Work out the finished part from the listing and answer in its coordinate system (mm). A direction names the side the tool comes from. Coordinates: 2 decimals unless noted, no trailing zeros. Order: outer loops, then holes, each group sorted by start corner. A loop starts at its lowest first (then second) coordinate and runs counter-clockwise, first axis right, second up. Notation, with made-up numbers: (29.25, -18) - (86.25, -18) arc R32 cw to (86.25, 20) - close; hole circle Ø2 at (76, 37.25). An arc over 180 degrees is marked (long way). Answer as a JSON object with one key per item and string values. Group by question number.
1) Find the intervals of material crossed by line 1 along X through (y, z) = (-14, -44); line 2 along X through (y, z) = (-0.5, -89.5); line 3 along Z through (x, y) = (51, 0), in increasing order.
2) Section A-A (z = -85) is taken. Count the separate pieces of the cut face and the enclosed holes in it, plus the area to 3 significant figures.
3) The mould has two halves that part along Z. Classify faces 6 (the face through (52, -8, -48)), 7 (the face through (66.667, 2, -86)), 8 (the face through (-70.388, -7.598, -95.496)): released by +Z, released by -Z, zero draft, split by the parting line, or undercut.
4) This flat-tipped pin is pushed along its axis until it touches: P1, Ø1.1, axis at x = -67.5, z = -25.5, coming from the -Y side. Where does it stop, or does it pass through?
5) Section D-D (y = -16) is taken. Give the vertices of the cut face in (x, z), plus the area to 3 significant figures.
6) Section B-B (x = 61) is taken. Give the vertices of the cut face in (y, z), plus the area to 3 significant figures.
7) A tool of negligible diameter and unlimited length cuts with its end or side. For faces 1 (the face through (-53.5, -9, -49)), 2 (the face through (71.814, -8, -49)), 3 (the face through (-52, -8, -48)), 4 (the face through (-66.667, 2, -12)), 5 (the face through (-70.311, -7.598, -1.426)), from which of +Z, -Z, +X, -X, +Y, -Y can it reach the whole face along a straight path? Write none if from no direction.
from build123d import *
from build123d.topology import SkipClean

# Parameters (mm, degrees)
CROQUIS1_W              = 114
CROQUIS1_H              = 34.2
SALIENTE_EXTRUIR1_DEPTH = 97
VACIADO1_T              = -5
SALIENTE_EXTRUIR2_DEPTH = 97
CORTAR_EXTRUIR1_REACH   = 128.031
CROQUIS3_W              = 13.814275766
CROQUIS3_H              = 40
REDONDEO2_R             = 5
CROQUIS6_W              = 12.3
CROQUIS6_H              = 10.4
CORTAR_EXTRUIR3_DEPTH   = 124.459670354
SALIENTE_EXTRUIR3_DEPTH = 97
CROQUIS8_W              = 13.814275766
CROQUIS8_H              = 40
CORTAR_EXTRUIR4_DEPTH   = 127.030661617
CROQUIS9_W              = 104
CROQUIS9_H              = 87
CORTAR_EXTRUIR5_DEPTH   = 10
CORTAR_EXTRUIR6_START   = -33.316303
CROQUIS11_W             = 1.5
CROQUIS11_H             = 39.999512223
CROQUIS11_H_2           = 40
CORTAR_EXTRUIR6_DEPTH   = 33.316303
CORTAR_EXTRUIR7_START   = -33.316303
CROQUIS13_W             = 15.314275766
CROQUIS13_H             = 4.5
CORTAR_EXTRUIR7_DEPTH   = 33.316303


with BuildPart() as part:
    # Croquis1 → Saliente-Extruir1 (new body)
    with BuildSketch(Plane.XY):
        with Locations((0, -8.9)):
            Rectangle(CROQUIS1_W, CROQUIS1_H)
    extrude(amount=-SALIENTE_EXTRUIR1_DEPTH)

    # Vaciado1
    vaciado1_openings = [part.faces().sort_by_distance(p)[0] for p in [
        (0, -26, -48.5),
    ]]
    offset(amount=VACIADO1_T, openings=vaciado1_openings, kind=Kind.INTERSECTION)

    # Croquis2 → Saliente-Extruir2 (add, through all)
    with BuildSketch(Plane(origin=(0, 0, -97), x_dir=(-1, 0, 0), z_dir=(0, 0, -1))):
        Polygon((71.814275766, 8.2), (67.33466189, 8.2), (67.33466189, -3.967393508), (57, -3.967393508), (57, -26), (67.33466189, -26), (71.814275766, -26), align=None)
        Polygon((-57, 8.2), (57, 8.2), (67.33466189, 8.2), (71.814275766, 8.2), (71.814275766, 10.296521374), (-71.814275766, 10.296521374), (-71.814275766, 8.2), (-67.33466189, 8.2), align=None)
        Polygon((-67.33466189, -3.967393508), (-67.33466189, 8.2), (-71.814275766, 8.2), (-71.814275766, -26), (-67.33466189, -26), (-57, -26), (-57, -3.967393508), align=None)
    extrude(amount=-SALIENTE_EXTRUIR2_DEPTH)

    # Croquis3 → Cortar-Extruir1 (cut, up to next)
    with BuildSketch(Plane.XZ.offset(26), mode=Mode.PRIVATE) as cortar_extruir1_sk1:
        with Locations((-61.907137883, -48.5)):
            Rectangle(CROQUIS3_W, CROQUIS3_H)
    cortar_extruir1_tool1 = extrude(cortar_extruir1_sk1.sketch, amount=-CORTAR_EXTRUIR1_REACH, mode=Mode.PRIVATE) & part.part
    # Croquis3 → Cortar-Extruir1 (cut, up to next)
    with BuildSketch(Plane.XZ.offset(26), mode=Mode.PRIVATE) as cortar_extruir1_sk2:
        with Locations((61.907137883, -48.5)):
            Rectangle(CROQUIS3_W, CROQUIS3_H)
    cortar_extruir1_tool2 = extrude(cortar_extruir1_sk2.sketch, amount=-CORTAR_EXTRUIR1_REACH, mode=Mode.PRIVATE) & part.part
    add(cortar_extruir1_tool1.solids().sort_by_distance((-61.907138, -26, -48.5))[0], mode=Mode.SUBTRACT)
    add(cortar_extruir1_tool2.solids().sort_by_distance((61.907138, -26, -48.5))[0], mode=Mode.SUBTRACT)

    # Redondeo2
    # the kernel refuses this fillet: 5 mm, written as the material it takes off along each edge
    with BuildSketch(Plane(origin=(71.814275766, -38.5, -97), x_dir=(0, 0, 1), z_dir=(0, 1, 0)), Plane(origin=(71.814275766, -38.5, 0), x_dir=(-1, 0, 0), z_dir=(0, 1, 0)), Plane(origin=(-71.814275766, 22.796521374, -97), x_dir=(0, 0, 1), z_dir=(0, -1, 0)), Plane(origin=(-71.814275766, 22.796521374, 0), x_dir=(1, 0, 0), z_dir=(0, -1, 0))) as redondeo2_piece_1:
        with BuildLine():
            CenterArc((REDONDEO2_R, -REDONDEO2_R), REDONDEO2_R, 90, 90)
            Line((0, -REDONDEO2_R), (0, 0))
            Line((0, 0), (REDONDEO2_R, 0))
        make_face()
    extrude(amount=61.296521374, mode=Mode.SUBTRACT)

    # Croquis6 → Cortar-Extruir3 (cut, through all)
    with BuildSketch(Plane(origin=(0, 0, -97), x_dir=(-1, 0, 0), z_dir=(0, 0, -1))):
        with Locations((-60.617330945, 2.116303246)):
            Rectangle(CROQUIS6_W, CROQUIS6_H)
        with Locations((60.617330945, 2.116303246)):
            Rectangle(CROQUIS6_W, CROQUIS6_H)
    extrude(amount=-CORTAR_EXTRUIR3_DEPTH, mode=Mode.SUBTRACT)

    # Croquis7 → Saliente-Extruir3 (add, through all)
    with BuildSketch(Plane(origin=(0, 0, -97), x_dir=(-1, 0, 0), z_dir=(0, 0, -1))):
        Polygon((57, 8.2), (57, 7.316303246), (66.667330945, 7.316303246), (66.667330945, -3.083696754), (57, -3.083696754), (57, -3.967393508), (66.814275766, -3.967393508), (67.33466189, -3.967393508), (67.33466189, 8.2), (66.814275766, 8.2), align=None)
        Polygon((-66.667330945, 7.32503221), (-57, 7.32503221), (-57, 8.2), (-66.814275766, 8.2), (-67.33466189, 8.2), (-67.33466189, -3.967393508), (-66.814275766, -3.967393508), (-57, -3.967393508), (-57, -3.083696754), (-66.667330945, -3.083696754), align=None)
    extrude(amount=-SALIENTE_EXTRUIR3_DEPTH)

    # Croquis8 → Cortar-Extruir4 (cut, through all)
    with BuildSketch(Plane(origin=(0, 10.296521374, 0), x_dir=(1, 0, 0), z_dir=(0, 1, 0))):
        with Locations((-61.907137883, 48.5)):
            Rectangle(CROQUIS8_W, CROQUIS8_H)
        with Locations((61.907137883, 48.5)):
            Rectangle(CROQUIS8_W, CROQUIS8_H)
    extrude(amount=-CORTAR_EXTRUIR4_DEPTH, mode=Mode.SUBTRACT)

    # Croquis9 → Cortar-Extruir5 (cut)
    with BuildSketch(Plane.XZ.offset(-3.2)):
        with Locations((0, -48.5)):
            Rectangle(CROQUIS9_W, CROQUIS9_H)
    extrude(amount=-CORTAR_EXTRUIR5_DEPTH, mode=Mode.SUBTRACT)

    # Croquis11 → Cortar-Extruir6 (cut)
    with SkipClean():  # the faces are left unmerged after this step: merging them gives an invalid solid
        with BuildSketch(Plane.XZ.offset(26).offset(CORTAR_EXTRUIR6_START)):
            with Locations((54.25, -48.499756112)):
                Rectangle(CROQUIS11_W, CROQUIS11_H)
            with Locations((-54.25, -48.5)):
                Rectangle(CROQUIS11_W, CROQUIS11_H_2)
        extrude(amount=CORTAR_EXTRUIR6_DEPTH, mode=Mode.SUBTRACT)

    # Croquis13 → Cortar-Extruir7 (cut)
    with BuildSketch(Plane.XZ.offset(26).offset(CORTAR_EXTRUIR7_START)):
        with Locations((-61.157137883, -26.25)):
            Rectangle(CROQUIS13_W, CROQUIS13_H)
        with Locations((-61.157137883, -70.75)):
            Rectangle(CROQUIS13_W, CROQUIS13_H)
        with Locations((61.157137883, -26.25)):
            Rectangle(CROQUIS13_W, CROQUIS13_H)
        with Locations((61.157137883, -70.749512223)):
            Rectangle(CROQUIS13_W, CROQUIS13_H)
    extrude(amount=CORTAR_EXTRUIR7_DEPTH, mode=Mode.SUBTRACT)


solid = part.part
Report:
{
 "1": {"line 1": "x = -71.81 to -68.81, -53.5 to -52, 52 to 53.5, 68.81 to 71.81", "line 2": "x = -71.81 to -66.67, -54.47 to -52, 52 to 54.47, 66.67 to 71.81", "line 3": "z = -97 to -92, -5 to 0"},
 "2": {"separate pieces": "2", "enclosed holes": "2", "area": "1,180 mm²"},
 "3": {"face 6": "undercut", "face 7": "zero draft", "face 8": "released by -Z"},
 "4": {"P1": "stops at y = 7.32"},
 "5": {"outline": "(-71.81, -92) arc R5 ccw to (-66.81, -97) - (66.81, -97) arc R5 ccw to (71.81, -92) - (71.81, -5) arc R5 ccw to (66.81, 0) - (-66.81, 0) arc R5 ccw to (-71.81, -5) - close; hole (-68.81, -73) - (-53.5, -73) - (-53.5, -24) - (-68.81, -24) - close; hole (-52, -92) - (52, -92) - (52, -5) - (-52, -5) - close; hole (53.5, -73) - (68.81, -73) - (68.81, -24) - (53.5, -24) - close", "area": "3,360 mm²"},
 "6": {"outline": "(-26, -97) - (-3.08, -97) - (-3.08, -73) - (-26, -73) - close; (-26, -24) - (-3.08, -24) - (-3.08, 0) - (-26, 0) - close; (7.33, -97) - (10.3, -97) - (10.3, -68.5) - (7.33, -68.5) - close; (7.33, -28.5) - (10.3, -28.5) - (10.3, 0) - (7.33, 0) - close", "area": "1,270 mm²"},
 "7": {"face 1": "-Y", "face 2": "+Z, -Z, +X, +Y, -Y", "face 3": "+Y, -Y", "face 4": "+Z, -Z", "face 5": "+Z, -X, +Y, -Y"}
}
